```python
from build123d import *

# Parameters (mm, degrees)
SKETCH1_W                = 155
SKETCH1_H                = 105
SKETCH1_W_2              = 125.476190476
SKETCH1_H_2              = 85
BOSS_EXTRUDE1_DEPTH      = 3
BOSS_EXTRUDE2_DEPTH      = 18.5
BOSS_EXTRUDE2_DEPTH_BACK = 3
SKETCH2_W                = 8
SKETCH2_H                = 105
BOSS_EXTRUDE3_DEPTH      = 18.5
BOSS_EXTRUDE3_DEPTH_BACK = 3
SKETCH3_W                = 30
SKETCH3_H                = 6
SKETCH4_W                = 25
SKETCH4_H                = 105
SKETCH4_W_2              = 30
SKETCH4_H_2              = 12
BOSS_EXTRUDE4_DEPTH      = 5
SKETCH5_R                = 12
SKETCH5_W                = 8.45267088
SKETCH5_H                = 74.460442491
SKETCH5_W_2              = 90.792338418
SKETCH5_H_2              = 7.04119429
CUT_EXTRUDE1_DEPTH       = 5
SKETCH7_R                = 3
CUT_EXTRUDE3_DEPTH       = 5
SKETCH8_W                = 40
SKETCH8_H                = 45
BOSS_EXTRUDE7_DEPTH      = 12
SKETCH10_W               = 34
SKETCH10_H               = 39
CUT_EXTRUDE4_DEPTH       = 9


with BuildPart() as part:
    # Sketch1 → Boss-Extrude1 (new body)
    # profile 1 of 2: a face of its own
    with BuildSketch(Plane(origin=(0, 0, 0), x_dir=(1, 0, 0), z_dir=(0, 1, 0))):
        Rectangle(SKETCH1_W, SKETCH1_H)
        Rectangle(SKETCH1_W_2, SKETCH1_H_2, mode=Mode.SUBTRACT)
    # profile 2 of 2: a face of its own
    with BuildSketch(Plane(origin=(0, 0, 0), x_dir=(1, 0, 0), z_dir=(0, 1, 0))):
        Polygon((62.738095238, 8), (22.507606796, 8), (36.015047402, 17.1502017), (62.738095238, 35.252911525), (62.738095238, 42.5), (52.040012251, 42.5), (29.28486966, 27.085225986), (8, 12.666443314), (8, 42.5), (-8, 42.5), (-8, 12.666443314), (-22.464140061, 22.464731742), (-52.040012251, 42.5), (-62.738095238, 42.5), (-62.738095238, 35.252911525), (-29.194317803, 12.529707456), (-22.507606796, 8), (-62.738095238, 8), (-62.738095238, -8), (-23.178437825, -8), (-62.738095238, -36.5), (-62.738095238, -42.5), (-52.040012251, -42.5), (-21.061503369, -21.514558499), (-8, -12.666443314), (-8, -42.5), (8, -42.5), (8, -12.666443314), (21.061503369, -21.514558499), (52.040012251, -42.5), (62.738095238, -42.5), (62.738095238, -35.252911525), (27.791681111, -11.579534213), (22.507606796, -8), (62.738095238, -8), align=None)
    extrude(amount=BOSS_EXTRUDE1_DEPTH)

    # Sketch2 → Boss-Extrude2 (add, two sides: drawn at the far end of the back side and taken through both)
    with BuildSketch(Plane(origin=(0, 3, 0), x_dir=(1, 0, 0), z_dir=(0, 1, 0)).offset(-BOSS_EXTRUDE2_DEPTH_BACK)):
        with Locations((-81.5, 0)):
            Rectangle(SKETCH2_W, SKETCH2_H)
        with Locations((81.5, 0)):
            Rectangle(SKETCH2_W, SKETCH2_H)
    extrude(amount=BOSS_EXTRUDE2_DEPTH + BOSS_EXTRUDE2_DEPTH_BACK)

    # Sketch3 → Boss-Extrude3 (add, two sides: drawn at the far end of the back side and taken through both)
    with BuildSketch(Plane(origin=(0, 3, 0), x_dir=(1, 0, 0), z_dir=(0, 1, 0)).offset(-BOSS_EXTRUDE3_DEPTH_BACK)):
        with Locations((0, -55.5)):
            Rectangle(SKETCH3_W, SKETCH3_H)
        with Locations((0, 55.5)):
            Rectangle(SKETCH3_W, SKETCH3_H)
    extrude(amount=BOSS_EXTRUDE3_DEPTH + BOSS_EXTRUDE3_DEPTH_BACK)

    # Sketch4 → Boss-Extrude4 (add)
    with BuildSketch(Plane(origin=(0, 21.5, 0), x_dir=(1, 0, 0), z_dir=(0, 1, 0))):
        with Locations((-65, 0)):
            Rectangle(SKETCH4_W, SKETCH4_H)
        with Locations((65, 0)):
            Rectangle(SKETCH4_W, SKETCH4_H)
        with Locations((0, 46.5)):
            Rectangle(SKETCH4_W_2, SKETCH4_H_2)
        with Locations((0, -46.5)):
            Rectangle(SKETCH4_W_2, SKETCH4_H_2)
    extrude(amount=-BOSS_EXTRUDE4_DEPTH)

    # Sketch5 → Cut-Extrude1 (cut)
    with BuildSketch(Plane(origin=(0, 3, 0), x_dir=(1, 0, 0), z_dir=(0, 1, 0))):
        Circle(SKETCH5_R)
        with Locations((-0.467592264, 5.065542336)):
            Rectangle(SKETCH5_W, SKETCH5_H)
        with Locations((1.005079981, -0.147085174)):
            Rectangle(SKETCH5_W_2, SKETCH5_H_2)
    extrude(amount=-CUT_EXTRUDE1_DEPTH, mode=Mode.SUBTRACT)

    # Sketch7 → Cut-Extrude3 (cut)
    with BuildSketch(Plane(origin=(0, 21.5, 0), x_dir=(1, 0, 0), z_dir=(0, 1, 0))):
        with Locations(Location((-61.471836621, 0, 0), (0, 0, 270))):
            Circle(SKETCH7_R)
        with Locations(Location((62.160596695, 0, 0), (0, 0, 270))):
            Circle(SKETCH7_R)
        with Locations(Location((-61.471836621, 34.395123429, 0), (0, 0, 270))):
            Circle(SKETCH7_R)
        with Locations(Location((-61.471836621, -33.490958607, 0), (0, 0, 270))):
            Circle(SKETCH7_R)
        with Locations(Location((62.160596695, 34.861702835, 0), (0, 0, 270))):
            Circle(SKETCH7_R)
        with Locations(Location((62.160596695, -33.490958607, 0), (0, 0, 270))):
            Circle(SKETCH7_R)
        with Locations(Location((0, -44.855499831, 0), (0, 0, 270))):
            Circle(SKETCH7_R)
        with Locations(Location((0, 46.060829961, 0), (0, 0, 270))):
            Circle(SKETCH7_R)
    extrude(amount=-CUT_EXTRUDE3_DEPTH, mode=Mode.SUBTRACT)

    # Sketch8 → Boss-Extrude7 (add)
    with BuildSketch(Plane(origin=(0, 3, 0), x_dir=(1, 0, 0), z_dir=(0, 1, 0))):
        Rectangle(SKETCH8_W, SKETCH8_H)
    extrude(amount=BOSS_EXTRUDE7_DEPTH)

    # Sketch10 → Cut-Extrude4 (cut)
    with BuildSketch(Plane(origin=(0, 15, 0), x_dir=(1, 0, 0), z_dir=(0, 1, 0))):
        Rectangle(SKETCH10_W, SKETCH10_H)
    extrude(amount=-CUT_EXTRUDE4_DEPTH, mode=Mode.SUBTRACT)


solid = part.part
```
Design review of the part built by this model. Coordinates are the model's own, in mm. A direction names the side the tool comes from. Give positions to 0.01 mm unless a question says otherwise; leave off trailing zeros. Loops run counter-clockwise (first coordinate to the right, second up) from the corner with the lowest first, then second, coordinate; pieces in that order, holes last. Notation, with made-up numbers: (-18, 34) -> (14, 34) arc R14 cw to (14, 60) -> close; hole circle Ø7 at (-28, 73). An arc over 180 degrees is marked (long way). Write each question's results on one line, items separated by ' | '.
Q1. The part is to be moulded in two halves that separate along Z. For faces 5 (the face through (0, 11, -58.5)), 6 (the face through (85.5, 11, 1)), 7 (the face through (-18, 15, 0)), say which applies: +Z half, -Z half, draft (parallel to the pull), parting line (faces both ways), or undercut.
Reply:
face 5: -Z half | face 6: draft | face 7: undercut
Q2. For pin 1 Ø0.9 at (x, y) = (51, 1.5) entering from +Z; pin 2 Ø12 at (x, z) = (3, -15) entering from +Y; pin 3 Ø2.5 at (x, y) = (-38.5, 1) entering from -Z, all flat-tipped, find the tip position at first contact; note any pin that passes through.
Reply:
pin 1: stops at z = 52.5 | pin 2: stops at y = 15 | pin 3: stops at z = -52.5
Q3. Wall thickness on L1, parallel to X at y = 3.25, z = 10; L2, parallel to Z at x = 14, y = 5.5; L3, parallel to Y at x = -56.5, z = -34.5: over which ranges is each line inside the solid? List them lowest first.
Reply:
L1: x = -85.5 to -77.5, -20 to 20, 77.5 to 85.5 | L2: z = -58.5 to -52.5, -22.5 to 22.5, 52.5 to 58.5 | L3: y = 0 to 3, 16.5 to 21.5
Q4. Take a section at B-B, the plane x = 0. Give the number of separate pieces and of enclosed holes in the cut face, plus the area to 3 significant figures.
Reply:
separate pieces: 5 | enclosed holes: 0 | area: 599 mm²
Q5. Take a section at A-A, the plane y = 9.5. Write out the cut boundary in (x, z), plus the area to 3 significant figures.
Reply:
outline: (-85.5, -52.5) -> (-77.5, -52.5) -> (-77.5, 52.5) -> (-85.5, 52.5) -> close; (-20, -22.5) -> (20, -22.5) -> (20, 22.5) -> (-20, 22.5) -> close; (-15, -58.5) -> (15, -58.5) -> (15, -52.5) -> (-15, -52.5) -> close; (-15, 52.5) -> (15, 52.5) -> (15, 58.5) -> (-15, 58.5) -> close; (77.5, -52.5) -> (85.5, -52.5) -> (85.5, 52.5) -> (77.5, 52.5) -> close; hole (-17, -19.5) -> (17, -19.5) -> (17, 19.5) -> (-17, 19.5) -> close | area: 2,510 mm²
Q6. Machinability: for faces 1 (the face through (0, 10, 52.5)), 2 (the face through (8.683, 1.521, -8.283)), 3 (the face through (-66.1, 2.8, 52.5)), 4 (the face through (17, 11, 0)), which of the approach directions +Z, -Z, +X, -X, +Y, -Y give a long, thin tool a straight path to every point of the face, cutting with its end or side? Answer none if there is none.
Reply:
face 1: none | face 2: -Y | face 3: +Z, -X, +Y, -Y | face 4: +Y
Q7. Take a section at D-D, the plane x = -49.5. Write out the cut boundary in (y, z), plus the area to 3 significant figures.
Reply:
outline: (0, -52.5) -> (3, -52.5) -> (3, -42.5) -> (0, -42.5) -> close; (0, -40.78) -> (3, -40.78) -> (3, -26.29) -> (0, -26.29) -> close; (0, -8) -> (3, -8) -> (3, 8) -> (0, 8) -> close; (0, 26.96) -> (3, 26.96) -> (3, 40.78) -> (0, 40.78) -> close; (0, 42.5) -> (3, 42.5) -> (3, 52.5) -> (0, 52.5) -> close | area: 193 mm²
